```python
from build123d import *

# Parameters (mm, degrees)
F1_DEPTH = 10
F3_D     = 6.6


with BuildPart() as f1:
    # F0 (on Front) → F1 (new body)
    with BuildSketch(Plane.XZ):
        with BuildLine():
            Line((0, 43.5), (0, 0))
            Line((0, 0), (15.4, 0))
            ThreePointArc((15.4, 0), (40, 24.6), (64.6, 0))
            Line((64.6, 0), (80, 0))
            Line((80, 0), (80, 43.5))
            Line((80, 43.5), (0, 43.5))
        make_face()
    extrude(amount=F1_DEPTH)

    # F3 (through all)
    with Locations(Plane.XY.offset(43.5)):
        with Locations((8, -5), (72, -5)):
            Hole(F3_D / 2)


solid = f1.part
```
Check sheet for the modelled part. Datum: model origin and axes. Units: mm. Give positions to 0.01 mm unless a question says otherwise; leave off trailing zeros. Order: outer loops, then holes, each group sorted by start corner. A loop starts at its lowest first (then second) coordinate and runs counter-clockwise, first axis right, second up. Notation, with made-up numbers: M 42,8 L 72,8 A3 cw 72,13 Z; hole C -29,73.5 d11. An arc over 180 degrees is marked long. Answer in a Markdown table with one row per item.
1) Release check for a two-part mould opening along Y. For faces 1 (the cylindrical face through (75.3, -4.9, 21.4)), 2 (the flat face through (39, -10, 27)), 3 (the flat face through (80, -5, 21)), 4 (the flat face through (39, 0, 27)) record: +Y half, -Y half, draft (parallel to the pull), parting line (faces both ways), or undercut.
Filled sheet:
| item | result |
|---|---|
| face 1 | undercut |
| face 2 | -Y half |
| face 3 | draft |
| face 4 | +Y half |
2) Cross-section at D-D, the plane y = -3.5. Enter the section's corners in (x, z).
Filled sheet:
| item | result |
|---|---|
| outline | M 0,0 L 5.06,0 L 5.06,43.5 L 0,43.5 Z; M 10.94,0 L 15.4,0 A24.6 cw 64.6,0 L 69.06,0 L 69.06,43.5 L 10.94,43.5 Z; M 74.94,0 L 80,0 L 80,43.5 L 74.94,43.5 Z |
3) Cross-section at A-A, the plane z = 10. Enter the section's corners in (x, y), plus the area to 3 significant figures.
Filled sheet:
| item | result |
|---|---|
| outline | M 0,-10 L 17.52,-10 L 17.52,0 L 0,0 Z; M 62.48,-10 L 80,-10 L 80,0 L 62.48,0 Z; hole C 8,-5 d6.6; hole C 72,-5 d6.6 |
| area | 282 mm2 |
4) Cross-section at B-B, the plane x = 72. Enter the section's corners in (y, z), plus the area to 3 significant figures.
Filled sheet:
| item | result |
|---|---|
| outline | M -10,0 L -8.3,0 L -8.3,43.5 L -10,43.5 Z; M -1.7,0 L 0,0 L 0,43.5 L -1.7,43.5 Z |
| area | 148 mm2 |
5) Cross-section at C-C, the plane z = 41.5. Enter the section's corners in (x, y).
Filled sheet:
| item | result |
|---|---|
| outline | M 0,-10 L 80,-10 L 80,0 L 0,0 Z; hole C 8,-5 d6.6; hole C 72,-5 d6.6 |
6) Thickness scan on L1, parallel to X at y = -6.25, z = 29.5; L2, parallel to Y at x = 8, z = 30; L3, parallel to X at y = -2.5, z = 25.5. Record the ranges inside material, lowest first. Write a range as [from, to].
Filled sheet:
| item | result |
|---|---|
| L1 | x = [0, 4.95], [11.05, 68.95], [75.05, 80] |
| L2 | y = [-10, -8.3], [-1.7, 0] |
| L3 | x = [0, 5.85], [10.15, 69.85], [74.15, 80] |
